The model under review builds one solid part; all positions refer to its coordinate system, in mm. A direction names the side the tool comes from. Round coordinates to 2 decimals unless told otherwise and drop trailing zeros. Loops run counter-clockwise (first coordinate to the right, second up) from the corner with the lowest first, then second, coordinate; pieces in that order, holes last. Notation, with made-up numbers: M -17,34.25 L -7,34.25 A34 cw -7,67.25 Z; hole C 22,23 d11. An arc over 180 degrees is marked long. One line per question, with ' | ' between items.
from build123d import *

# Parameters (mm, degrees)
SKETCH1_W               = 120.396
SKETCH1_H               = 203.2
BOSS_EXTRUDE1_DEPTH     = 6.35
CUT_EXTRUDE1_START      = -7.35
SKETCH2_W               = 25.4
SKETCH2_H               = 25.4
CUT_EXTRUDE1_DEPTH      = 8.35
MIRROR2_START           = -7.35
MIRROR2_COPY_1_SKETCH_W = 25.4
MIRROR2_COPY_1_SKETCH_H = 25.4
MIRROR2_COPY_1_DEPTH    = 8.35
SKETCH3_W               = 44.45
SKETCH3_H               = 45.72
SKETCH3_H_2             = 53.34
CUT_EXTRUDE2_DEPTH      = 7.35


with BuildPart() as part:
    # Sketch1 → Boss-Extrude1 (new body)
    with BuildSketch(Plane(origin=(0, 0, 0), x_dir=(1, 0, 0), z_dir=(0, 1, 0))):
        Rectangle(SKETCH1_W, SKETCH1_H)
    extrude(amount=BOSS_EXTRUDE1_DEPTH)

    # Sketch2 → Cut-Extrude1 (cut)
    with BuildSketch(Plane(origin=(0, 6.35, 0), x_dir=(1, 0, 0), z_dir=(0, 1, 0)).offset(CUT_EXTRUDE1_START)):
        with Locations((-41.148, 76.2)):
            Rectangle(SKETCH2_W, SKETCH2_H)
    cut_extrude1 = extrude(amount=CUT_EXTRUDE1_DEPTH, mode=Mode.SUBTRACT)

    # Mirror1: Cut-Extrude1 across plane
    add(cut_extrude1.mirror(Plane.XY), mode=Mode.SUBTRACT)

    # Mirror2: Cut-Extrude1 across plane
    add(cut_extrude1.mirror(Plane(origin=(0, 0, 0), x_dir=(0, 0, 1), z_dir=(1, 0, 0))), mode=Mode.SUBTRACT)

    # Mirror2 copy 1 sketch → Mirror2 copy 1 (cut)
    with BuildSketch(Plane(origin=(0, 6.35, 0), x_dir=(-1, 0, 0), z_dir=(0, 1, 0)).offset(MIRROR2_START)):
        with Locations((-41.148, 76.2)):
            Rectangle(MIRROR2_COPY_1_SKETCH_W, MIRROR2_COPY_1_SKETCH_H)
    extrude(amount=MIRROR2_COPY_1_DEPTH, mode=Mode.SUBTRACT)

    # Sketch3 → Cut-Extrude2 (cut, through all)
    with BuildSketch(Plane(origin=(0, 6.35, 0), x_dir=(1, 0, 0), z_dir=(0, 1, 0))):
        with Locations((0, -78.74)):
            Rectangle(SKETCH3_W, SKETCH3_H)
        with Locations((0, 74.93)):
            Rectangle(SKETCH3_W, SKETCH3_H_2)
    extrude(amount=-CUT_EXTRUDE2_DEPTH, mode=Mode.SUBTRACT)


solid = part.part
1) Add section D-D on z = -58.5. State the section outline as (x, y) points (3 decimals).
Output values:
outline: M -60.198,0 L -22.225,0 L -22.225,6.35 L -60.198,6.35 Z; M 22.225,0 L 60.198,0 L 60.198,6.35 L 22.225,6.35 Z
2) Mouldability with a two-part tool opening along X and no side actions: class faces 4 (the flat face through (-1, 0, -1)), 5 (the flat face through (28.448, 3, -76)) as +X half, -X half, draft (parallel to the pull), parting line (faces both ways), or undercut.
Output values:
face 4: draft | face 5: undercut
3) Machinability: for faces 1 (the flat face through (0, 3, 55.88)), 2 (the flat face through (22.225, 3, -75)), 3 (the flat face through (-53.848, 3, 76)), which of the approach directions +Z, -Z, +X, -X, +Y, -Y give a long, thin tool a straight path to every point of the face, cutting with its end or side? Answer none if there is none.
Output values:
face 1: +Z, +Y, -Y | face 2: -Z, +Y, -Y | face 3: +Y, -Y
4) Add section C-C on z = 82. State the section outline as (x, y) points (3 decimals).
Output values:
outline: M -60.198,0 L -53.848,0 L -53.848,6.35 L -60.198,6.35 Z; M -28.448,0 L -22.225,0 L -22.225,6.35 L -28.448,6.35 Z; M 22.225,0 L 28.448,0 L 28.448,6.35 L 22.225,6.35 Z; M 53.848,0 L 60.198,0 L 60.198,6.35 L 53.848,6.35 Z
5) Add section B-B on y = 3. State the section outline as (x, z) points (3 decimals), then the cut area to 3 significant figures.
Output values:
outline: M -60.198,-101.6 L -22.225,-101.6 L -22.225,-48.26 L 22.225,-48.26 L 22.225,-101.6 L 60.198,-101.6 L 60.198,101.6 L 22.225,101.6 L 22.225,55.88 L -22.225,55.88 L -22.225,101.6 L -60.198,101.6 Z; hole M -53.848,-88.9 L -28.448,-88.9 L -28.448,-63.5 L -53.848,-63.5 Z; hole M -53.848,63.5 L -28.448,63.5 L -28.448,88.9 L -53.848,88.9 Z; hole M 28.448,-88.9 L 53.848,-88.9 L 53.848,-63.5 L 28.448,-63.5 Z; hole M 28.448,63.5 L 53.848,63.5 L 53.848,88.9 L 28.448,88.9 Z | area: 17,500 mm²
6) Insertion check: P1, Ø5, axis at x = 11, z = 33, coming from the -Y side; P2, Ø2, axis at x = 9, y = 1.5, coming from the -Z side. Each pin has a flat end and moves straight along its axis. Give the tip position at first contact, or say it passes through.
Output values:
P1: stops at y = 0 | P2: stops at z = -48.26
7) For line 1 (Z direction, x = -43.5, y = 3.5); line 2 (X direction, y = 3.75, z = 77) (3 decimals); line 3 (X direction, y = 4, z = -60) (3 decimals), list the stretches that pass through material, from the lowest coordinate up.
Output values:
line 1: z = -101.6 to -88.9, -63.5 to 63.5, 88.9 to 101.6 | line 2: x = -60.198 to -53.848, -28.448 to -22.225, 22.225 to 28.448, 53.848 to 60.198 | line 3: x = -60.198 to -22.225, 22.225 to 60.198
8) Add section A-A on x = -37. State the section outline as (y, z) points, then the cut area to 3 significant figures.
Output values:
outline: M 0,-101.6 L 6.35,-101.6 L 6.35,-88.9 L 0,-88.9 Z; M 0,-63.5 L 6.35,-63.5 L 6.35,63.5 L 0,63.5 Z; M 0,88.9 L 6.35,88.9 L 6.35,101.6 L 0,101.6 Z | area: 968 mm²
